Geometry: final body of the model. Coordinates: model frame, mm. A direction names the side the tool comes from. Give positions to 0.01 mm unless a question says otherwise; leave off trailing zeros. Write each loop counter-clockwise with the first axis right and the second up, starting at its lowest first coordinate (ties: lowest second). Pieces come first, ordered by that corner, then holes.
Q1. Reachability of faces 5 (the face through (0, 0, 12.5)), 6 (the face through (-0.54, 2.44, 5.92)), 7 (the face through (5.4, 0, 17.5)), 8 (the face through (-5.4, 0, 7.5)) from +Z, -Z, +X, -X, +Y, -Y: full face, straight path, thin tool, end or side. Return the list, or none.
Q2. Line query: L1, parallel to X at y = 0, z = 15.75; L2, parallel to Y at x = 0, z = 6.75. Output: solid intervals per line, ascending.
Q3. Cut plane C-C on x = 0. Return the cut outline in (y, z), plus the area to 3 significant figures.
Q4. Cut plane D-D on z = 16. Return the cut outline in (x, y).
Q5. Cut plane B-B on z = 5.25. Return the cut outline in (x, y).
Q6. Pin query (flat end, axial travel): pin 1 (1 mm diameter, centred on y = 1, z = 20, fed in from +X); pin 2 (2 mm diameter, centred on y = 0, z = 14, fed in from -X); pin 3 (3 mm diameter, centred on x = 0, y = 0, fed in from +Z). Return the tip coordinate at first contact, or that it passes through.
Q7. Cut plane A-A on y = 0. Return the cut outline in (x, z), plus the area to 3 significant figures.
Q8. Draft query along Y for faces 1 (the face through (0.54, 2.44, 18.58)), 2 (the face through (3, 0, 0)), 3 (the face through (0, 0, 12)), 4 (the face through (-4.76, 3.65, 12.08)). Return one class per face: pulls with the +Y half, pulls with the -Y half, needs draft (parallel to the pull), parting line crosses it, or undercut.
Autodesk Fusion 360 part; units mm, degrees
sketch "Esquisse1" plane through (0, 0, 0) normal (0, 0, 1) x (1, 0, 0)
  circle A0 centre (0, 0) radius 6
  dimension "d1" = 12
extrude "Extrusion1" add sketch "Esquisse1" along normal blind 24.5
sketch "Esquisse2" plane through (0, 0, 24.5) normal (0, 0, 1) x (-1, 0, 0)
  circle A0 centre (0, 0) radius 6
  circle A1 centre (0, 0) radius 2.5
  dimension "d5" = 5
extrude "Extrusion2" cut sketch "Esquisse2" against normal blind 12 contours A1
sketch "Esquisse3" plane through (0, 0, 0) normal (0, 0, -1) x (1, 0, 0)
  circle A0 centre (0, 0) radius 6
  circle A1 centre (0, 0) radius 2.5
  dimension "d8" = 5
extrude "Extrusion3" cut sketch "Esquisse3" against normal blind 12 contours A1
sketch "Esquisse4" plane through (0, 0, 24.5) normal (0, 0, 1) x (-1, 0, 0)
  circle A0 centre (0, 0) radius 2.5
  circle A1 centre (0, 0) radius 6
  line L0 (5, 8) -> (-5, 8)
  line L1 (-5, 8) -> (-5, -7.4606)
  line L2 (-5, -7.4606) -> (5, -7.4606)
  line L3 (5, -7.4606) -> (5, 8)
  dimension "d11" = 5
  dimension "d12" = 10
extrude "Extrusion4" cut sketch "Esquisse4" against normal blind 10 from surface at -7 contours A1 L3 | A1 L1
Data:
1. face 5: +Z
1. face 6: -Z
1. face 7: +X, +Y, -Y
1. face 8: -X, +Y, -Y
2. L1: x = -5 to -2.5, 2.5 to 5
2. L2: y = -6 to -2.5, 2.5 to 6
3. outline: (-6, 0) - (-2.5, 0) - (-2.5, 12) - (2.5, 12) - (2.5, 0) - (6, 0) - (6, 24.5) - (2.5, 24.5) - (2.5, 12.5) - (-2.5, 12.5) - (-2.5, 24.5) - (-6, 24.5) - close
3. area: 174 mm2
4. outline: (-5, -3.32) arc R6 ccw to (5, -3.32) - (5, 3.32) arc R6 ccw to (-5, 3.32) - close; hole circle Ø5 at (0, 0)
5. outline: circle Ø12 at (0, 0); hole circle Ø5 at (0, 0)
6. pin 1: stops at x = 5.98
6. pin 2: stops at x = -5
6. pin 3: stops at z = 12.5
7. outline: (-6, 0) - (-2.5, 0) - (-2.5, 12) - (2.5, 12) - (2.5, 0) - (6, 0) - (6, 7.5) - (5, 7.5) - (5, 17.5) - (6, 17.5) - (6, 24.5) - (2.5, 24.5) - (2.5, 12.5) - (-2.5, 12.5) - (-2.5, 24.5) - (-6, 24.5) - (-6, 17.5) - (-5, 17.5) - (-5, 7.5) - (-6, 7.5) - close
7. area: 154 mm2
8. face 1: undercut
8. face 2: needs draft
8. face 3: undercut
8. face 4: parting line crosses it
